Autodesk Fusion 360 part; units mm, degrees
sketch "Esquisse1" plane through (0, 0, 0) normal (0, 0, 1) x (1, 0, 0)
  line L0 (0, 0) -> (53.1, 0)
  line L1 (53.1, 0) -> (53.1, 66.2)
  line L2 (0, 66.2) -> (0, 0)
  line L3 (40.9, 0) -> (49.9, 0)
  line L4 (49.9, 0) -> (49.9, -5.2)
  line L5 (49.9, -5.2) -> (40.9, -5.2)
  line L6 (40.9, -5.2) -> (40.9, 0)
  line L7 (11.5, 0) -> (18.8, 0)
  line L8 (18.8, 0) -> (18.8, -1.2)
  line L9 (18.8, -1.2) -> (11.5, -1.2)
  line L10 (11.5, -1.2) -> (11.5, 0)
  line L11 (53.1, 66.2) -> (50.8, 66.2) construction
  line L12 (50.8, 66.2) -> (48.7068, 69)
  line L13 (48.7068, 69) -> (14.6068, 69)
  line L14 (12.1, 66.2) -> (14.6068, 69)
  line L15 (53.1, 66.2) -> (50.8, 66.2)
  line L16 (12.1, 66.2) -> (0, 66.2)
  line L17 (40.9, 0) -> (49.9, 0)
  line L18 (11.5, 0) -> (18.8, 0)
  line L19 (0, 33.1) -> (53.1, 33.1) construction
  line L20 (26.55, 0) -> (26.55, 33.1) construction
  line L21 (0, 66.2) -> (0, 68.7) construction
  line L22 (0, 68.7) -> (53.1, 68.7) construction
  line L23 (53.1, 68.7) -> (53.1, 66.2) construction
  line L24 (-3, 72) -> (56.1, 72)
  line L25 (56.1, 72) -> (56.1, -3)
  line L26 (56.1, -3) -> (-3, -3)
  line L27 (-3, -3) -> (-3, 72)
  line L28 (-6, 75) -> (59.1, 75)
  line L29 (59.1, 75) -> (59.1, -5)
  line L30 (59.1, -5) -> (-6, -5)
  line L31 (-6, -5) -> (-6, 75)
  line L32 (26.55, 75) -> (26.55, -5) construction
  line L33 (11.5, -1.2) -> (11.5, -5)
  line L34 (18.8, -1.2) -> (18.8, -5)
  line L35 (15.15, 0) -> (15.15, -5) construction
  line L36 (9.55, 0) -> (20.75, 0)
  line L37 (20.75, 0) -> (20.75, -5)
  line L38 (20.75, -5) -> (9.55, -5)
  line L39 (9.55, -5) -> (9.55, 0)
  line L40 (15.15, 0) -> (15.15, -5) construction
  line L41 (-3, -3) -> (-6, -3)
  line L42 (56.1, -3) -> (59.1, -3)
  dimension "d1" = 66.2
  dimension "d13" = 53.1
  dimension "d14" = 3.2
  dimension "d15" = 9
  dimension "d16" = 5.2
  dimension "d17" = 11.5
  dimension "d18" = 7.3
  dimension "d19" = 1.2
  dimension "d21" = 2.3
  dimension "d22" = 38.7
  dimension "d25" = 34.1
  dimension "d43" = 3
  dimension "d44" = 3
  dimension "d45" = 3
  dimension "d46" = 3
  dimension "d47" = 3
  dimension "d48" = 3
  dimension "d52" = 11.2
extrude "Extrusion6" add sketch "Esquisse1" along normal blind 1 contours L0 L1 L2 L3 L7 L12 L13 L14 L15 L16 L17 L18 L36
extrude "Extrusion7" add sketch "Esquisse1" along normal blind 5.5 draft 1 contours L0 L1 L2 L4 L12 L13 L14 L15 L16 L24 L25 L26 L27 L39 | L0 L6 L26 L37
extrude "Extrusion8" add sketch "Esquisse1" along normal blind 20 contours L24 L25 L27 L28 L29 L31 L41 L42
extrude "Extrusion9" add sketch "Esquisse1" along normal blind 4.5 contours L0 L10 L26 L33 L36 L39 | L0 L7 L8 L9 L10 L18 L36 | L26 L30 L33 L38 L39 | L0 L8 L26 L34 L36 L37 | L9 L26 L33 L34 | L26 L30 L33 L34 L38 | L26 L30 L34 L37 L38 | L0 L3 L4 L6 L17 L26 | L4 L6 L26 L30
extrude "Extrusion10" add sketch "Esquisse1" along normal blind 14.8 contours L26 L30 L31 L39 L41 | L6 L26 L30 L37 | L4 L26 L29 L30 L42
sketch "Esquisse2" plane through (-3, 0, 0) normal (1, 0, 0) x (0, 1, 0)
  line L0 (-3, 5.5) -> (72, 5.5)
  line L1 (72, 5.5) -> (72, 20)
  line L2 (72, 20) -> (-3, 20)
  line L3 (-3, 20) -> (-3, 14.8)
  line L4 (-3, 14.8) -> (-3, 5.5)
  line L5 (-3, 20) -> (75, 20) construction
  line L6 (-3, 18) -> (72.5, 18)
  line L7 (72.5, 18) -> (72.5, 13.8)
  line L8 (72.5, 13.8) -> (-3, 13.8)
  line L9 (-3, 13.8) -> (-3, 18)
  dimension "d65" = 2
  dimension "d66" = 4.2
  dimension "d67" = 75.5
extrude "Extrusion11" cut sketch "Esquisse2" against normal blind 1.5 contours L1 L3 L4 L6 L8 L9
sketch "Esquisse3" plane through (56.1, 0, 0) normal (-1, 0, 0) x (0, -1, 0)
  line L0 (-72, 5.5) -> (3, 5.5)
  line L1 (3, 5.5) -> (3, 14.8)
  line L2 (3, 14.8) -> (3, 20)
  line L3 (3, 20) -> (-72, 20)
  line L4 (-72, 20) -> (-72, 5.5)
  line L5 (-72, 20) -> (3, 20) construction
  line L6 (-72, 18) -> (3, 18)
  line L7 (3, 18) -> (3, 13.8)
  line L8 (3, 13.8) -> (-72, 13.8)
  line L9 (-72, 13.8) -> (-72, 18)
  dimension "d70" = 4.2
  dimension "d71" = 2
extrude "Extrusion12" cut sketch "Esquisse3" against normal blind 1.5 contours L1 L2 L4 L6 L7 L8 L9
sketch "Esquisse4" plane through (0, 72, 0) normal (0, -1, 0) x (1, 0, 0)
  line L0 (-3, 5.5) -> (56.1, 5.5)
  line L1 (56.1, 5.5) -> (56.1, 13.8)
  line L2 (56.1, 13.8) -> (57.6, 13.8)
  line L3 (57.6, 13.8) -> (57.6, 18)
  line L4 (57.6, 18) -> (56.1, 18)
  line L5 (56.1, 18) -> (56.1, 20)
  line L6 (56.1, 20) -> (-3, 20)
  line L7 (-3, 20) -> (-3, 18)
  line L8 (-3, 18) -> (-4.5, 18)
  line L9 (-4.5, 18) -> (-4.5, 13.8)
  line L10 (-4.5, 13.8) -> (-3, 13.8)
  line L11 (-3, 13.8) -> (-3, 5.5)
  line L12 (-4.5, 18) -> (57.6, 18)
  line L13 (57.6, 18) -> (57.6, 13.8)
  line L14 (57.6, 13.8) -> (-4.5, 13.8)
  line L15 (-4.5, 13.8) -> (-4.5, 18)
extrude "Extrusion13" add 2 faces at (43.9262, -1.0262, 4.5) (16.9905, -1.0262, 4.5) along direction (0, 0, 1) blind 0.8
sketch "Esquisse5" plane through (0, -3, 0) normal (0, 1, 0) x (-1, 0, 0)
  line L0 (-40.9, 5.5) -> (-20.75, 5.5)
  line L1 (-20.75, 5.5) -> (-20.75, 14.8)
  line L2 (-20.75, 14.8) -> (-40.9, 14.8)
  line L3 (-40.9, 14.8) -> (-40.9, 5.5)
  line L4 (-59.8312, 14.8) -> (5.1812, 14.8) construction
  line L5 (-50, 16) -> (-40.9, 16) construction
  line L6 (-20.75, 13.5) -> (-9.5, 13.5) construction
  line L7 (-40.9, 5.5) -> (-51, 5.5) construction
  line L8 (-51, 5.5) -> (-20.75, 5.5) construction
  line L9 (-9.284, 5.5) -> (-20.75, 5.5) construction
  line L10 (-50, 16) -> (-40.9, 16)
  line L11 (-40.9, 16) -> (-40.9, 14.8)
  line L12 (-40.9, 14.8) -> (-50, 14.8)
  line L13 (-50, 14.8) -> (-50, 16)
  line L14 (-20.75, 14.8) -> (-9.5, 14.8)
  line L15 (-9.5, 14.8) -> (-9.5, 13.5)
  line L16 (-9.5, 13.5) -> (-20.75, 13.5)
  line L17 (-20.75, 13.5) -> (-20.75, 14.8)
  line L18 (-27.325, 14.8) -> (-34.325, 14.8)
  line L19 (-34.325, 14.8) -> (-34.325, 10.8)
  line L20 (-34.325, 10.8) -> (-27.325, 10.8)
  line L21 (-27.325, 10.8) -> (-27.325, 14.8)
  line L22 (-20.75, 14.8) -> (-40.9, 14.8) construction
  line L23 (-40.9, 14.8) -> (-40.9, 5.5) construction
  line L24 (-40.9, 5.5) -> (-20.75, 5.5) construction
  line L25 (-20.75, 5.5) -> (-20.75, 14.8) construction
  line L26 (-30.825, 14.8) -> (-30.825, 10.8) construction
  line L27 (-30.825, 14.8) -> (-30.825, 5.5) construction
  dimension "d76" = 10.5
  dimension "d78" = 8
  dimension "d81" = 7
  dimension "d82" = 4
extrude "Extrusion14" add sketch "Esquisse5" against normal blind 2 contours L10 L11 L12 L13 | L1 L14 L15 L16 L17
extrude "Extrusion16" cut sketch "Esquisse5" against normal blind 2 contours L2 L18 L19 L20 L21
extrude "Extrusion17" cut sketch "Esquisse4" against normal blind 1 contours L2 L3 L4 L8 L9 L10 L12 L13 L14 L15
extrude "Extrusion19" cut 1 faces at (46.9667, -3.6667, 16) along direction (0, 0, -1) blind 3
equation "d1 = longc1"
equation "longc1 = longueur Carte"
equation "largc1 = largueur Carte"
equation "diffdepH = 2.5 mm"
equation "epchar = 11 mm"
equation "depconn = 1.2 mm"
equation "depchar = 5.2 mm"
equation "larchar = 9 mm"
equation "larconn = 7.3 mm"
equation "distborconn = 11.5 mm"
equation "distborchar = 3.2 mm"
equation "diffdepD = 2.3 mm"
equation "d13 = largc1"
equation "d14 = distborchar"
equation "d15 = larchar"
equation "d16 = depchar"
equation "d17 = distborconn"
equation "d18 = larconn"
equation "d19 = depconn"
equation "largdep = 34.2 mm"
equation "d21 = diffdepD"
equation "epC = 4.5 mm"
equation "epconn = 2.5 mm"
equation "diffCB = espace entre bordure et carte"
equation "d43 = diffCB"
equation "d44 = diffCB"
equation "d45 = diffCB"
equation "d46 = diffCB"
equation "d47 = epB"
equation "d48 = epB"
equation "epB = 3 mm"
equation "Lpu = largeur de l'embout USB-c"
equation "Hpu = Hauteur de l'embout USB-c"
equation "d52 = Lpu"
equation "d55 = 1 mm + epC"
equation "HB = Hauteur Boite"
equation "epV = 3.2 mm"
equation "d59 = HB"
equation "d61 = epC"
equation "d63 = HB - 2 mm - epV"
equation "d66 = epV + 1 mm"
equation "d67 = 78.000001 mm - 2.5 mm"
equation "d70 = epV + 1 mm"
equation "d76 = HC"
equation "HC = hauteur del'embout chargeur"
equation "d78 = Hpu"
equation "longpin = 3 mm"
Verification items for the finished model (mm, model axes). A direction names the side the tool comes from. Give positions to 0.01 mm unless a question says otherwise; leave off trailing zeros. Loops run counter-clockwise (first coordinate to the right, second up) from the corner with the lowest first, then second, coordinate; pieces in that order, holes last.
1. Material ranges on probe 1 along X at (y, z) = (65.5, 12.5); probe 2 along X at (y, z) = (3.5, 5); probe 3 along Y at (x, z) = (27, 12.5), recorded low to high.
Derived:
probe 1: x = -6 to -3, 56.1 to 59.1
probe 2: x = -6 to 0.09, 53.01 to 59.1
probe 3: y = -5 to -3, 72 to 75
2. Cross-section at D-D on z = 4.25. Record the cut outline in (x, y), and give its area (3 significant figures).
Derived:
outline: (-6, -5) - (59.1, -5) - (59.1, 75) - (-6, 75) - close; hole (0.07, 0.07) - (9.62, 0.07) - (9.62, 0) - (20.68, 0) - (20.68, 0.07) - (40.97, 0.07) - (40.97, 0) - (49.83, 0) - (49.83, 0.07) - (53.03, 0.07) - (53.03, 66.13) - (50.76, 66.13) - (48.67, 68.93) - (14.64, 68.93) - (12.13, 66.13) - (0.07, 66.13) - close
area: 1,610 mm2
3. Go/stop test with flat-tipped pins: P1, Ø1, axis at x = 50.5, y = 21.5, coming from the +Z side; P2, Ø4, axis at x = 45, y = -2.5, coming from the +Z side; P3, Ø2.5, axis at x = 57, z = 17.5, coming from the -Y side; P4, Ø10, axis at x = 18.5, y = 44.5, coming from the -Z side. Record where each tip stops, or that it passes through.
Derived:
P1: stops at z = 1
P2: stops at z = 5.3
P3: stops at y = -3
P4: stops at z = 0
4. Cross-section at C-C on x = 33. Record the cut outline in (y, z), and give its area (3 significant figures).
Derived:
outline: (-5, 0) - (75, 0) - (75, 20) - (72, 20) - (72, 18) - (73, 18) - (73, 13.8) - (72, 13.8) - (72, 5.5) - (68.9, 5.5) - (68.98, 1) - (0.02, 1) - (0.1, 5.5) - (-3, 5.5) - (-3, 10.8) - (-5, 10.8) - close
area: 180 mm2
5. Cross-section at A-A on z = 8. Record the cut outline in (x, y).
Derived:
outline: (-6, -5) - (9.55, -5) - (9.55, -3) - (-3, -3) - (-3, 72) - (56.1, 72) - (56.1, -3) - (49.9, -3) - (49.9, -5) - (59.1, -5) - (59.1, 75) - (-6, 75) - close; (20.75, -5) - (40.9, -5) - (40.9, -3) - (20.75, -3) - close
6. Release check for a two-part mould opening along Z. For faces 1 (the flat face through (56.3, 35.2, 18)), 2 (the flat face through (40.9, -4, 10)) record: +Z half, -Z half, draft (parallel to the pull), parting line (faces both ways), or undercut.
Derived:
face 1: undercut
face 2: draft
7. Cross-section at B-B on y = 64. Record the cut outline in (x, z), and give its area (3 significant figures).
Derived:
outline: (-6, 0) - (59.1, 0) - (59.1, 20) - (56.1, 20) - (56.1, 18) - (57.6, 18) - (57.6, 13.8) - (56.1, 13.8) - (56.1, 5.5) - (53, 5.5) - (53.08, 1) - (0.02, 1) - (0.1, 5.5) - (-3, 5.5) - (-3, 13.8) - (-4.5, 13.8) - (-4.5, 18) - (-3, 18) - (-3, 20) - (-6, 20) - close
area: 194 mm2
8. Tool access check on faces 3 (the flat face through (20.75, -4, 9)), 4 (the flat face through (26, 72, 10)), 5 (the flat face through (-5, -3, 18)). Record the directions out of +Z, -Z, +X, -X, +Y, -Y that give a thin tool (end or side, any length) a straight path to the whole face; none if there is none.
Derived:
face 3: -Y
face 4: +Z
face 5: +Z, +X, -X, -Y
